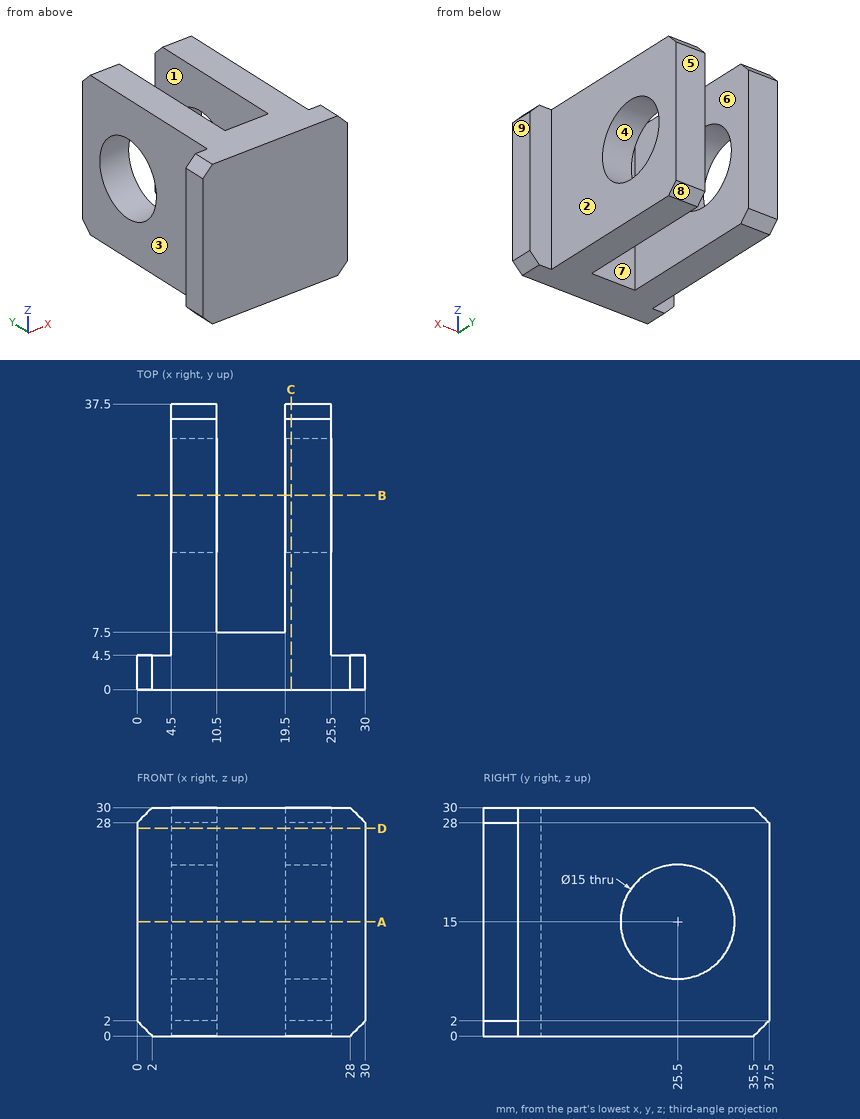
Could you check a few things on this drawing? It's one solid part, dimensions in mm from its lowest x, y, z. A direction names the side the tool comes from. Coordinates: 2 decimals unless noted, no trailing zeros. Order: outer loops, then holes, each group sorted by start corner. A loop starts at its lowest first (then second) coordinate and runs counter-clockwise, first axis right, second up. Notation, with made-up numbers: (73, 15.25) -> (121, 15.25) arc R14 ccw to (121, 24.25) -> close; hole circle Ø3 at (-27, -37.75). An arc over 180 degrees is marked (long way). One line per item, written item: value. Start each with the question number.
1) Imagine slicing it at A-A on z = 15. List the corners of the cut face in (x, y) for me, plus the area to 3 significant figures.
2) I'm going to push flat-ended pins straight in: pin 1 (4 mm diameter, centred on y = 17, z = 4, fed in from +X); pin 2 (1 mm diameter, centred on y = 6, z = 15.5, fed in from -X); pin 3 (3.5 mm diameter, centred on x = 2.5, z = 15.5, fed in from +Y). Where does each tip first touch, or does it pass through?
3) Imagine slicing it at B-B on y = 25.5. List the corners of the cut face in (x, z) for me.
4) Imagine slicing it at D-D on z = 27.25. List the corners of the cut face in (x, y) for me, plus the area to 3 significant figures.
5) Imagine slicing it at C-C on x = 20.25. List the corners of the cut face in (y, z) for me.
6) Which directions (+Z, -Z, +X, -X, +Y, -Y) give clear straight access to the entire face, cutting with the end or side of a thin tool? Please do the marked faces 1, 2, 3, 4 and 5.
7) If I drill on L1, parallel to X at y = 29.5, z = 6; L2, parallel to Y at x = 7.8, z = 15; L3, parallel to Y at x = 17, z = 27.75, over which ranges is the centre line in solid material (lowest first)? Write a range as [from, to].
8) We'd pull the mould along X, two halves only. Please class the marked faces 6, 7, 8 and 9: +X half, -X half, draft (parallel to the pull), parting line (faces both ways), or undercut.
Answer list:
1. outline: (0, 0) -> (30, 0) -> (30, 4.5) -> (25.5, 4.5) -> (25.5, 18) -> (19.5, 18) -> (19.5, 7.5) -> (10.5, 7.5) -> (10.5, 18) -> (4.5, 18) -> (4.5, 4.5) -> (0, 4.5) -> close; (4.5, 33) -> (10.5, 33) -> (10.5, 37.5) -> (4.5, 37.5) -> close; (19.5, 33) -> (25.5, 33) -> (25.5, 37.5) -> (19.5, 37.5) -> close
1. area: 378 mm2
2. pin 1: stops at x = 25.5
2. pin 2: stops at x = 4.5
2. pin 3: stops at y = 4.5
3. outline: (4.5, 0) -> (10.5, 0) -> (10.5, 7.5) -> (4.5, 7.5) -> close; (4.5, 22.5) -> (10.5, 22.5) -> (10.5, 30) -> (4.5, 30) -> close; (19.5, 0) -> (25.5, 0) -> (25.5, 7.5) -> (19.5, 7.5) -> close; (19.5, 22.5) -> (25.5, 22.5) -> (25.5, 30) -> (19.5, 30) -> close
4. outline: (0, 0) -> (30, 0) -> (30, 4.5) -> (25.5, 4.5) -> (25.5, 37.5) -> (19.5, 37.5) -> (19.5, 7.5) -> (10.5, 7.5) -> (10.5, 37.5) -> (4.5, 37.5) -> (4.5, 4.5) -> (0, 4.5) -> close
4. area: 558 mm2
5. outline: (0, 0) -> (35.5, 0) -> (37.5, 2) -> (37.5, 28) -> (35.5, 30) -> (0, 30) -> close; hole circle Ø15 at (25.5, 15)
6. face 1: +Z, -Z, +Y
6. face 2: +Z, -Z, +X, +Y
6. face 3: +Z, -Z, -X, +Y
6. face 4: +X, -X
6. face 5: +Z, -Z, +X, -X, +Y
7. L1: x = [4.5, 10.5], [19.5, 25.5]
7. L2: y = [0, 18], [33, 37.5]
7. L3: y = [0, 7.5]
8. face 6: undercut
8. face 7: undercut
8. face 8: draft
8. face 9: +X half
